```python
from build123d import *

# Parameters (mm, degrees)
F0_W      = 41.91
F0_H      = 19.05
F1_DEPTH  = 8.128
F3_DEPTH  = 41.911
F4_W      = 0.508
F4_H      = 2.54
F5_DEPTH  = 41.911
F8_SIZE   = 0.762
F10_DEPTH = 8.128
F11_R     = 3.81
F12_DEPTH = 8.128
F14_D     = 4.5
F14_DEPTH = 38.1
F14_TIP   = 1.3519363928
F15_R     = 0.762


with BuildPart() as f1:
    # F0 (on Top) → F1 (new body)
    with BuildSketch(Plane.XY):
        Rectangle(F0_W, F0_H)
    extrude(amount=F1_DEPTH)

    # F2 (on face) → F3 (cut, through all)
    with BuildSketch(Plane.YZ.offset(20.955)):
        Polygon((-9.525, 5.588), (0, 8.128), (-9.525, 8.128), align=None)
        Polygon((-4.7625, 0), (-9.525, 2.54), (-9.525, 0), align=None)
    extrude(amount=-F3_DEPTH, mode=Mode.SUBTRACT)

    # F4 (on face) → F5 (cut, through all)
    with BuildSketch(Plane.YZ.offset(20.955)):
        with Locations((-9.525, 4.064)):
            Rectangle(F4_W, F4_H)
    extrude(amount=-F5_DEPTH, mode=Mode.SUBTRACT)

    # F6 (on Right) → F7 (revolve)
    with BuildSketch(Plane.YZ):
        with BuildLine():
            Line((0, 5.08), (30.353, 5.08))
            Line((30.353, 5.08), (30.353, 8.89))
            Line((30.353, 8.89), (20.828, 8.89))
            Line((20.828, 8.89), (20.051436257, 9.983367576))
            Line((20.051436257, 9.983367576), (5.6547833958, 9.983367576))
            ThreePointArc((5.6547833958, 9.983367576), (2.6790917075, 9.507672027), (0, 8.128))
            Line((0, 8.128), (0, 5.08))
        make_face()
    revolve(axis=Axis((0, 15.1765, 5.08), (0, 1, 0)))

    # F8
    f8_edges = [f1.edges().sort_by_distance(p)[0] for p in [
        (0, 30.353, 1.27),
    ]]
    chamfer(f8_edges, length=F8_SIZE)

    # F9 (on Top) → F10 (join, through all)
    with BuildSketch(Plane.XY):
        Polygon((-3.8409256157, 9.525), (3.8409256157, 9.525), (4.903367576, 9.525), (4.903367576, 20.051436257), (-4.903367576, 20.051436257), (-4.903367576, 9.525), align=None)
        Polygon((4.903367576, 20.051436257), (4.903367576, 9.525), (20.955, 9.525), align=None)
        Polygon((-20.955, 9.525), (-4.903367576, 9.525), (-4.903367576, 20.051436257), align=None)
    extrude(amount=F10_DEPTH)

    # F11 (on face) → F12 (join, through all)
    with BuildSketch(Plane.XY.offset(8.128)):
        with Locations((13.97, 11.557)):
            Circle(F11_R)
        with Locations((-13.97, 11.557)):
            Circle(F11_R)
    extrude(amount=-F12_DEPTH)

    # F14
    with Locations(Plane.XY.offset(8.128)):
        with Locations((-13.97, 11.557), (13.97, 11.557)):
            Hole(F14_D / 2, depth=F14_DEPTH)
            with Locations((0, 0, -(F14_DEPTH + F14_TIP / 2))):  # 118° drill point
                Cone(0, F14_D / 2, F14_TIP, mode=Mode.SUBTRACT)

    # F15
    f15_edges = [f1.edges().sort_by_distance(p)[0] for p in [
        (20.955, 9.525, 4.064),
        (-20.955, 9.525, 4.064),
    ]]
    fillet(f15_edges, radius=F15_R)


solid = f1.part
```
Geometry check sheet. Reference: the model listing, model coordinates, mm. A direction names the side the tool comes from. Coordinates: 2 decimals unless noted, no trailing zeros. Write each loop counter-clockwise with the first axis right and the second up, starting at its lowest first coordinate (ties: lowest second). Pieces come first, ordered by that corner, then holes. Notation, with made-up numbers: M -38,31 L -14,31 A9 ccw -14,45 Z; hole C 13.25,63.25 d5. An arc over 180 degrees is marked long. Use one line per item in the form item = value. Start each with the question number.
1) Section check B-B on y = 22. Enter the section's corners in (x, z), and give its area (3 significant figures).
2) Go/stop test with flat-tipped pins: pin 1 Ø3 at (y, z) = (17.5, 8) entering from -X; pin 2 Ø16 at (x, y) = (9, 6.5) entering from +Z; pin 3 Ø0.5 at (x, z) = (4, 6.5) entering from +Y. Record where each tip stops, or that it passes through.
3) Thickness scan on probe 1 along Y at (x, z) = (13.97, 3.5); probe 2 along X at (y, z) = (12, 5); probe 3 along Z at (x, y) = (-2.5, 19). Record the ranges inside material, lowest first. Write a range as from..to.
4) Set-up check for faces 1 (the flat face through (0, 5, 0)), 2 (the flat face through (4.6, 20.051, 7.4)), 3 (the flat face through (-4.6, 20.051, 7.4)): record each of +Z, -Z, +X, -X, +Y, -Y from which the full face is reachable in a straight line by a thin tool's end or side.
5) Release check for a two-part mould opening along Y. For faces 4 (the cylindrical face through (-16.05, 10.7, 4.01)), 5 (the flat face through (-19.18, 10.69, 4.01)), 6 (the cylindrical face through (-1.46, 25.15, 8.6)) record: pulls with the +Y half, pulls with the -Y half, needs draft (parallel to the pull), parting line crosses it, or undercut.
Responses:
q1.outline = C 0,5.08 d7.62
q1.area = 45.6 mm2
q2.pin_1 = -11.08
q2.pin_2 = 9.88
q2.pin_3 = 20.7
q3.probe_1 = -9.27..9.31, 13.81..15.37
q3.probe_2 = -17.75..-16.18, -11.76..11.76, 16.18..17.75
q3.probe_3 = 0..9.3
q4.face_1 = -Z, +X, -X, +Y, -Y
q4.face_2 = +Z, +X, +Y
q4.face_3 = +Z, -X, +Y
q5.face_4 = undercut
q5.face_5 = pulls with the +Y half
q5.face_6 = needs draft
